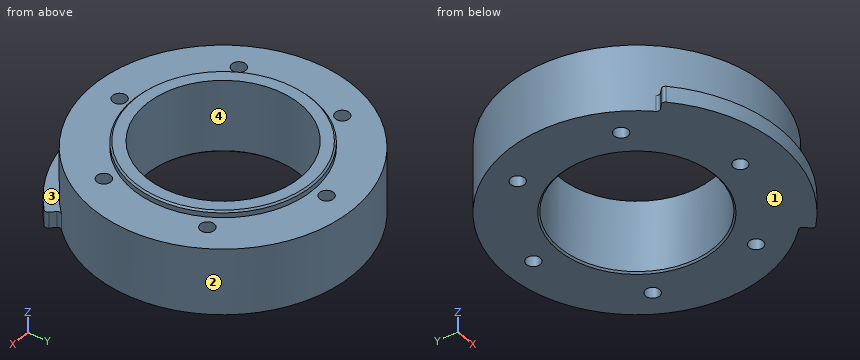
Autodesk Inventor part; units mm, degrees
ref_plane "YZ Plane" through (0, 0, 0) normal (1, 0, 0) x (0, 1, 0)
ref_plane "XZ Plane" through (0, 0, 0) normal (0, 1, 0) x (-1, 0, 0)
ref_plane "XY Plane" through (0, 0, 0) normal (0, 0, 1) x (1, 0, 0)
sketch "スケッチ1" plane through (0, 0, 0) normal (1, 0, 0) x (0, 1, 0)
  line L0 (40.5, 0) -> (24, 0)
  line L1 (24, 0) -> (24, -20.7)
  line L2 (24, -20.7) -> (40.5, -20.7)
  line L3 (40.5, -20.7) -> (40.5, 0)
  line L4 (0, -24.84) -> (0, 4.14)
  point P0 (0, 0)
  dimension "d0" = 24
  dimension "d2" = 40.5
  dimension "d3" = 20.7
revolve "回転1" add sketch "スケッチ1" angle 360 about axis through (0, 0, -10) along (0, 0, 1)
sketch "スケッチ2" plane through (0, 0, 0) normal (0, 0, 1) x (1, 0, 0)
  circle A0 centre (0, 0) radius 32
  point P0 (0, 32)
  point P1 (-27.7128, 16)
  point P2 (-27.7128, -16)
  point P3 (0, -32)
  point P4 (27.7128, -16)
  point P5 (27.7128, 16)
  dimension "d5" = 64
  dimension "d8" = 360
hole "穴1" at (0, 32, 0) at (-27.7128, 16, 0) at (-27.7128, -16, 0) at (0, -32, 0) at (27.7128, -16, 0) at (27.7128, 16, 0) direction (0, 0, -1) diameter 4.3 end through all
sketch "スケッチ3" plane through (0, 0, -20.7) normal (0, 0, 1) x (1, 0, 0)
  circle A0 centre (0, 0) radius 40.5
  circle A1 centre (0, 0) radius 44.5
  line L0 (0, 0) -> (-31.4663, -31.4663)
  line L1 (0, 0) -> (31.4663, -31.4663)
  line L2 (0, 62.3) -> (0, -62.3)
  point P0 (-28.6378, -28.6378)
  point P1 (28.6378, -28.6378)
  point P2 (19.901, -39.802)
  dimension "d17" = 4
  dimension "d23" = 45
  dimension "d24" = 45
extrude "押し出し1" add sketch "スケッチ3" along normal blind 5 contours L1 A1 L2 A0 | A0 L2 A1 L0 picked at (28.2757, -32.3682) picked at (-28.2757, -32.3682)
fillet "フィレット1" radius 1 4 edges at (-31.4663, -31.4663, -18.2) (31.4663, -31.4663, -18.2) (28.6378, -28.6378, -18.2) (-28.6378, -28.6378, -18.2)
sketch "スケッチ5" plane through (0, 0, 0) normal (0, 0, 1) x (1, 0, 0)
  circle A0 centre (0, 0) radius 24
  circle A1 centre (0, 0) radius 28
  dimension "d28" = 4
extrude "押し出し3" add sketch "スケッチ5" along normal blind 2
chamfer "面取り1" distance 0.5 angle 45 1 edges at (-28, 0, 2)
chamfer "面取り2" distance 0.5 angle 45 1 edges at (0, -24, -20.7)
properties part number "unit-base7" material "ABS プラスチック"
Read the model definition and answer for the solid it produces. Units are mm, in the model's axes. Face numbers are marked on the shaded views. A direction names the side the tool comes from. Coordinates: 2 decimals unless noted, no trailing zeros. Write each loop counter-clockwise with the first axis right and the second up, starting at its lowest first coordinate (ties: lowest second). Pieces come first, ordered by that corner, then holes. Notation, with made-up numbers: M 1,-15.75 L 15,-15.75 A5 ccw 15,-11.75 Z; hole C 15,19 d10. An arc over 180 degrees is marked long. Use a Markdown table: item, result.
Q1. Each of these flat-tipped pins is pushed along its axis until it touches: pin 1 Ø4 at (x, z) = (-24, -2) entering from +Y; pin 2 Ø1 at (y, z) = (21.5, -17.5) entering from +X; pin 3 Ø5 at (x, y) = (0, 32) entering from -Z; pin 4 Ø3 at (y, z) = (-4.5, -12) entering from +X. Where does it stop, or does it pass through?
Answer block:
| item | result |
|---|---|
| pin 1 | stops at y = 34 |
| pin 2 | stops at x = 34.63 |
| pin 3 | stops at z = -20.7 |
| pin 4 | stops at x = 40.39 |
Q2. The part is cut by section A-A, the plane z = -4.75. Write down the section's boundary in (x, y).
Answer block:
| item | result |
|---|---|
| outline | C 0,0 d81; hole C -27.71,-16 d4.3; hole C -27.71,16 d4.3; hole C 0,0 d48; hole C 0,-32 d4.3; hole C 0,32 d4.3; hole C 27.71,-16 d4.3; hole C 27.71,16 d4.3 |
Q3. Determine the mould class of the marked faces 3 and 4 for opening direction Y: released by +Y, released by -Y, zero draft, split by the parting line, or undercut.
Answer block:
| item | result |
|---|---|
| face 3 | zero draft |
| face 4 | undercut |
Q4. The part is cut by section C-C, the plane x = -33.5. Write down the section's boundary in (y, z), then the cut area to 3 significant figures.
Answer block:
| item | result |
|---|---|
| outline | M -22.76,-20.7 L 22.76,-20.7 L 22.76,0 L -22.76,0 Z |
| area | 942 mm2 |
Q5. Which of the six approach directions +Z, -Z, +X, -X, +Y, -Y give full straight-line access (tool end or side, diameter ignored) to the marked faces 1 and 2?
Answer block:
| item | result |
|---|---|
| face 1 | -Z, +X, -X, +Y, -Y |
| face 2 | +Z |
Q6. Straight lines are drawn through the part: L1, parallel to Y at x = 0, z = -8.5; L2, parallel to X at y = -16, z = -13.75; L3, parallel to Y at x = -28, z = -1. For each, find the intervals that lie inside material, in ascending order. Write a range as [from, to].
Answer block:
| item | result |
|---|---|
| L1 | y = [-40.5, -34.15], [-29.85, -24], [24, 29.85], [34.15, 40.5] |
| L2 | x = [-37.21, -29.86], [-25.56, -17.89], [17.89, 25.56], [29.86, 37.21] |
| L3 | y = [-29.26, -18.13], [-13.87, 13.87], [18.13, 29.26] |
